```python
from build123d import *

# Parameters (mm, degrees)
SKETCH1_R                   = 18.5
SKETCH1_R_2                 = 11.5
BOSS_EXTRUDE1_DEPTH         = 4
SKETCH2_R                   = 2
BOSS_EXTRUDE2_DEPTH         = 6
TAP_DRILL_FOR_M3X0_5_TAP1_D = 2.5
CUT_EXTRUDE1_DEPTH          = 10
FILLET1_R                   = 5
SKETCH6_R                   = 3.5
SKETCH6_R_2                 = 2
BOSS_EXTRUDE3_DEPTH         = 0.7


with BuildPart() as part:
    # Sketch1 → Boss-Extrude1 (new body)
    with BuildSketch(Plane.XY):
        Circle(SKETCH1_R)
        Circle(SKETCH1_R_2, mode=Mode.SUBTRACT)
    extrude(amount=BOSS_EXTRUDE1_DEPTH)

    # Sketch2 → Boss-Extrude2 (add)
    with BuildSketch(Plane.XY.offset(4)):
        with Locations((0, 15)):
            Circle(SKETCH2_R)
        with Locations((12.990381057, -7.5)):
            Circle(SKETCH2_R)
        with Locations((-12.990381057, -7.5)):
            Circle(SKETCH2_R)
    extrude(amount=BOSS_EXTRUDE2_DEPTH)

    # Tap Drill for M3x0.5 Tap1 (through all)
    with Locations(Plane(origin=(0, 15, 10), x_dir=(1, 0, 0), z_dir=(0, 0, 1))):
        with Locations((0, 0), (12.990381057, -22.5), (-12.990381057, -22.5)):
            Hole(TAP_DRILL_FOR_M3X0_5_TAP1_D / 2)

    # Sketch5 → Cut-Extrude1 (cut)
    with BuildSketch(Plane.XY.offset(4)):
        with BuildLine():
            ThreePointArc((0, 18.5), (2.615259707, 17.326030238), (3.476098947, 14.591666667))
            ThreePointArc((3.476098947, 14.591666667), (12.990381057, 7.5), (14.37480349, -4.285443339))
            ThreePointArc((14.37480349, -4.285443339), (16.312412175, -6.398133741), (16.021470006, -9.249999937))
            ThreePointArc((16.021470006, -9.249999937), (16.021469952, 9.250000031), (0, 18.5))
        make_face()
        with BuildLine():
            ThreePointArc((-3.476098947, 14.591666667), (-2.615259707, 17.326030238), (0, 18.5))
            ThreePointArc((0, 18.5), (-16.021469952, 9.250000031), (-16.021470006, -9.249999937))
            ThreePointArc((-16.021470006, -9.249999937), (-16.312412175, -6.398133741), (-14.37480349, -4.285443339))
            ThreePointArc((-14.37480349, -4.285443339), (-12.990381057, 7.5), (-3.476098947, 14.591666667))
        make_face()
        with BuildLine():
            ThreePointArc((-10.898704543, -10.306223327), (-13.697152515, -10.927896455), (-16.021470006, -9.249999937))
            ThreePointArc((-16.021470006, -9.249999937), (0, -18.5), (16.021470006, -9.249999937))
            ThreePointArc((16.021470006, -9.249999937), (13.697152515, -10.927896455), (10.898704543, -10.306223327))
            ThreePointArc((10.898704543, -10.306223327), (0, -15), (-10.898704543, -10.306223327))
        make_face()
    extrude(amount=-CUT_EXTRUDE1_DEPTH, mode=Mode.SUBTRACT)

    # Fillet1
    fillet1_edges = [part.edges().sort_by_distance(p)[0] for p in [
        (-3.476098947, 14.591666667, 2),
        (-14.37480349, -4.285443339, 2),
        (14.37480349, -4.285443339, 2),
        (3.476098947, 14.591666667, 2),
        (-10.898704543, -10.306223327, 2),
        (10.898704543, -10.306223327, 2),
    ]]
    fillet(fillet1_edges, radius=FILLET1_R)

    # Sketch6 → Boss-Extrude3 (add)
    with BuildSketch(Plane.XY.offset(4)):
        with Locations((-12.990381057, -7.5)):
            Circle(SKETCH6_R)
        with Locations((-12.990381057, -7.5)):
            Circle(SKETCH6_R_2, mode=Mode.SUBTRACT)
        with Locations((0, 15)):
            Circle(SKETCH6_R)
        with Locations((0, 15)):
            Circle(SKETCH6_R_2, mode=Mode.SUBTRACT)
        with Locations((12.990381057, -7.5)):
            Circle(SKETCH6_R)
        with Locations((12.990381057, -7.5)):
            Circle(SKETCH6_R_2, mode=Mode.SUBTRACT)
    extrude(amount=BOSS_EXTRUDE3_DEPTH)


solid = part.part
```
CAD build for the part. Positions are in the model's coordinates, mm. A direction names the side the tool comes from. Coordinates: 2 decimals unless noted, no trailing zeros. Write each loop counter-clockwise with the first axis right and the second up, starting at its lowest first coordinate (ties: lowest second). Pieces come first, ordered by that corner, then holes.
(1) Flat gauge pins, fed straight in: pin 1 (5 mm diameter, centred on x = 10.5, y = 7, fed in from +Z); pin 2 (8 mm diameter, centred on x = -5, y = 10.5, fed in from +Z); pin 3 (2 mm diameter, centred on x = -12, z = 6, fed in from -Y). Where does each tip first touch, or does it go through?
(2) Cut at C-C, the plane x = -13. List the corners of the cut face in (y, z), and give its area (3 significant figures).
(3) 3-axis set-ups, long thin cutter, end or side, ignore diameter. For faces 1 (the face through (0, 17, 7)), 2 (the face through (1, 16, 10)): which of +Z, -Z, +X, -X, +Y, -Y reach the whole face in a straight line?
(4) Cut at B-B, the plane y = 5.5. List the corners of the cut face in (x, z), and give its area (3 significant figures).
(5) Cut at D-D, the plane y = -7.5. List the corners of the cut face in (x, z), and give its area (3 significant figures).
(6) Cut at A-A, the plane z = 8. List the corners of the cut face in (x, y), and give its area (3 significant figures).
(7) Drill centre lines: probe 1 along Y at (x, z) = (0, 1.55); probe 2 along X at (y, z) = (0, 2.7); probe 3 along X at (y, z) = (-7, 6). Where is each one in solid material? Low to high.
Geometry says:
1. pin 1: stops at z = 4
1. pin 2: stops at z = 4.7
1. pin 3: stops at y = -9.5
2. outline: (-11, 0) - (-8.75, 0) - (-8.75, 10) - (-9.5, 10) - (-9.5, 4.7) - (-11, 4.7) - close; (-6.25, 0) - (7.48, 0) - (7.48, 4) - (-4, 4) - (-4, 4.7) - (-5.5, 4.7) - (-5.5, 10) - (-6.25, 10) - close
2. area: 75.0 mm2
3. face 1: +Z
3. face 2: +Z, +X, -X, +Y, -Y
4. outline: (-13.96, 0) - (-10.1, 0) - (-10.1, 4) - (-13.96, 4) - close; (10.1, 0) - (13.96, 0) - (13.96, 4) - (10.1, 4) - close
4. area: 30.8 mm2
5. outline: (-16.49, 0) - (-14.24, 0) - (-14.24, 10) - (-14.99, 10) - (-14.99, 4.7) - (-16.49, 4.7) - close; (-11.74, 0) - (-8.72, 0) - (-8.72, 4) - (-9.49, 4) - (-9.49, 4.7) - (-10.99, 4.7) - (-10.99, 10) - (-11.74, 10) - close; (8.72, 0) - (11.74, 0) - (11.74, 10) - (10.99, 10) - (10.99, 4.7) - (9.49, 4.7) - (9.49, 4) - (8.72, 4) - close; (14.24, 0) - (16.49, 0) - (16.49, 4.7) - (14.99, 4.7) - (14.99, 10) - (14.24, 10) - close
5. area: 64.4 mm2
6. outline: circle Ø4 at (-12.99, -7.5); circle Ø4 at (0, 15); circle Ø4 at (12.99, -7.5); hole circle Ø2.5 at (-12.99, -7.5); hole circle Ø2.5 at (0, 15); hole circle Ø2.5 at (12.99, -7.5)
6. area: 23.0 mm2
7. probe 1: y = -15 to -11.5, 11.5 to 13.75, 16.25 to 18.5
7. probe 2: x = -15 to -11.5, 11.5 to 15
7. probe 3: x = -14.93 to -14.14, -11.84 to -11.05, 11.05 to 11.84, 14.14 to 14.93
